Design review of the part shown in the three views and the two pictorial views. Dimensions are in mm from the part's minimum x, y and z. A direction names the side the tool comes from. Give positions to 0.01 mm unless a question says otherwise; leave off trailing zeros. Loops run counter-clockwise (first coordinate to the right, second up) from the corner with the lowest first, then second, coordinate; pieces in that order, holes last. Notation, with made-up numbers: (32, 63) -> (65, 63) arc R25 cw to (65, 77) -> close; hole circle Ø6 at (0.5, 31.25). An arc over 180 degrees is marked (long way). Use CSV: the item, a comma, the result in double quotes. Start each with the question number.
Item 1: For the marked faces 4, 5 and 6, list the 3-axis set-ups (+Z, -Z, +X, -X, +Y, -Y) from which the entire face can be reached by the end or side of a thin tool; tool diameter is ignored.
Item 2: We need section D-D (y = 22.5). State the section outline as (x, z) points.
Item 3: We need section B-B (x = 35). State the section outline as (y, z) points.
Item 4: We need section C-C (z = 40.5). State the section outline as (x, y) points.
Item 5: We need section A-A (y = 35). State the section outline as (x, z) points, plus the area to 3 significant figures.
Item 6: The part is to be moulded in two halves that separate along X. For the marked faces 1, 2 and 3, say which applies: +X half, -X half, draft (parallel to the pull), parting line (faces both ways), or undercut.
Item 7: Clearance check with flat-ended pins moving along their axes: pin 1 (4.5 mm diameter, centred on x = 13.35, y = 22.5, fed in from +Z); pin 2 (6.5 mm diameter, centred on x = 35, y = 60, fed in from -Z); pin 3 (8 mm diameter, centred on y = 54, z = 17.5, fed in from +X); pin 4 (24 mm diameter, centred on x = 35, y = 35, fed in from +Z). State where each tip first meets the part, or that it passes through.
Item 8: Wall thickness on line 1 along Y through (x, z) = (35, 36); line 2 along X through (y, z) = (22, 21) (1 decimal); line 3 along Z through (x, y) = (8, 33): over which ranges is each line inside the solid? List them lowest first. Write a range as from..to.
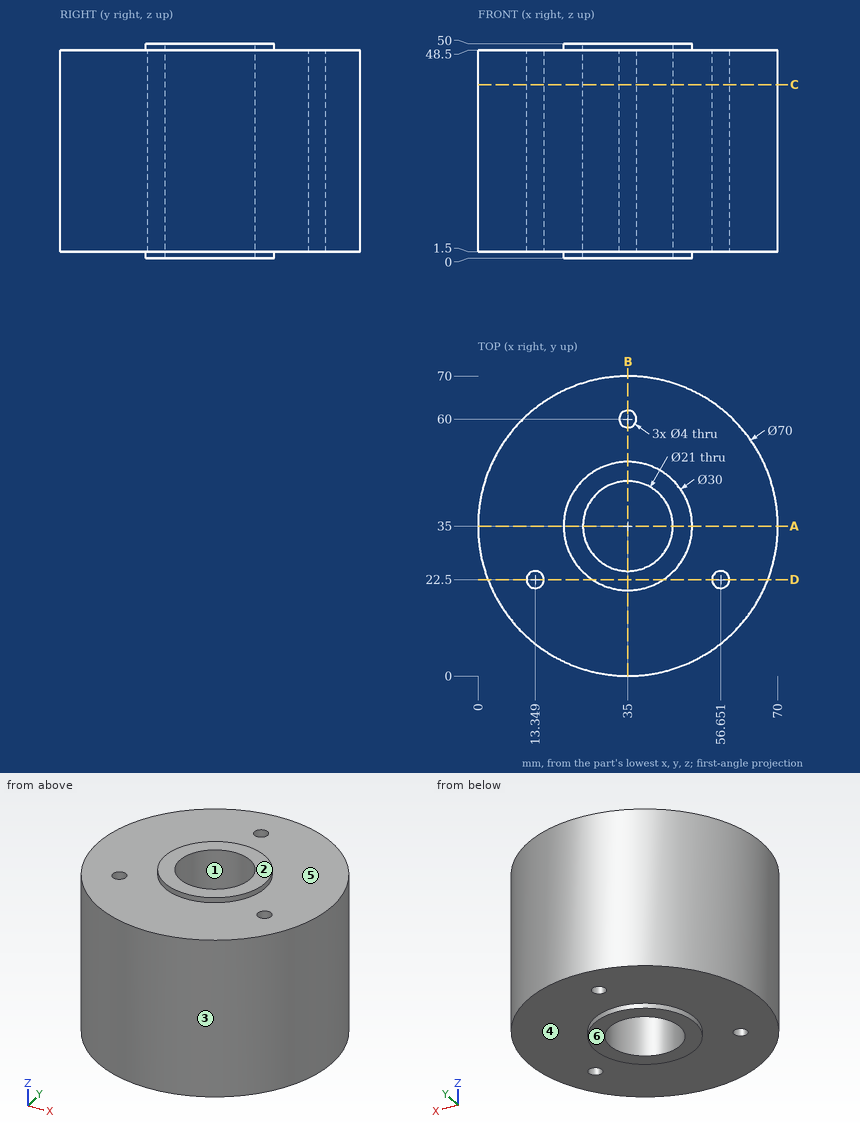
Results found:
1,face 4,"-Z"
1,face 5,"+Z"
1,face 6,"-Z, +X, -X, +Y, -Y"
2,outline,"(2.31, 1.5) -> (11.35, 1.5) -> (11.35, 48.5) -> (2.31, 48.5) -> close; (15.35, 1.5) -> (26.71, 1.5) -> (26.71, 0) -> (43.29, 0) -> (43.29, 1.5) -> (54.65, 1.5) -> (54.65, 48.5) -> (43.29, 48.5) -> (43.29, 50) -> (26.71, 50) -> (26.71, 48.5) -> (15.35, 48.5) -> close; (58.65, 1.5) -> (67.69, 1.5) -> (67.69, 48.5) -> (58.65, 48.5) -> close"
3,outline,"(0, 1.5) -> (20, 1.5) -> (20, 0) -> (24.5, 0) -> (24.5, 50) -> (20, 50) -> (20, 48.5) -> (0, 48.5) -> close; (45.5, 0) -> (50, 0) -> (50, 1.5) -> (58, 1.5) -> (58, 48.5) -> (50, 48.5) -> (50, 50) -> (45.5, 50) -> close; (62, 1.5) -> (70, 1.5) -> (70, 48.5) -> (62, 48.5) -> close"
4,outline,"circle Ø70 at (35, 35); hole circle Ø4 at (13.35, 22.5); hole circle Ø21 at (35, 35); hole circle Ø4 at (35, 60); hole circle Ø4 at (56.65, 22.5)"
5,outline,"(0, 1.5) -> (20, 1.5) -> (20, 0) -> (24.5, 0) -> (24.5, 50) -> (20, 50) -> (20, 48.5) -> (0, 48.5) -> close; (45.5, 0) -> (50, 0) -> (50, 1.5) -> (70, 1.5) -> (70, 48.5) -> (50, 48.5) -> (50, 50) -> (45.5, 50) -> close"
5,area,"2,330 mm²"
6,face 1,"undercut"
6,face 2,"draft"
6,face 3,"parting line"
7,pin 1,"z = 48.5"
7,pin 2,"z = 1.5"
7,pin 3,"x = 66.62"
7,pin 4,"z = 50"
8,line 1,"0..24.5, 45.5..58, 62..70"
8,line 2,"2.5..11.4, 15.3..54.7, 58.6..67.5"
8,line 3,"1.5..48.5"
